Geometry: final body of the model. Coordinates: model frame, mm. Give positions to 0.01 mm unless a question says otherwise; leave off trailing zeros. Write each loop counter-clockwise with the first axis right and the second up, starting at its lowest first coordinate (ties: lowest second). Pieces come first, ordered by that corner, then holes.
Q1. Pin query (flat end, axial travel): pin 1 (3 mm diameter, centred on x = 216.51, y = 75, fed in from +Z); pin 2 (1 mm diameter, centred on y = 81, z = 48, fed in from +X). Return the tip coordinate at first contact, or that it passes through.
Q2. Line query: L1, parallel to Y at x = 215, z = 46.55; L2, parallel to X at y = 75.5, z = 47.15; L3, parallel to Y at x = 207, z = 47. Output: solid intervals per line, ascending.
Q3. Draft query along X for faces 1 (the face through (234.19, 72.19, 47.3)), 2 (the face through (215.49, 76.6, 47.3)), 3 (the face through (244.56, 39.81, 47.3)). Return one class per face: pulls with the +X half, pulls with the -X half, needs draft (parallel to the pull), parting line crosses it, or undercut.
Q4. Cut plane B-B on y = 56. Return the cut outline in (x, z), plus the area to 3 significant figures.
Q5. Cut plane C-C on x = 209. Return the cut outline in (y, z), plus the area to 3 significant figures.
```python
from build123d import *

# Parameters (mm, degrees)
ESQUISSE1_R        = 1.902389191
BOSS_EXTRU_1_DEPTH = 3


with BuildPart() as part:
    # Esquisse1 → Boss.-Extru.1 (new body)
    with BuildSketch(Plane(origin=(0, 0, 48.781012584), x_dir=(-1, 0, 0), z_dir=(0, 0, -1))):
        with BuildLine():
            Line((-246.569633903, 56.844858091), (-221.455699093, 87.978285117))
            Line((-221.455699093, 87.978285117), (-202.775642878, 72.909924232))
            Line((-202.775642878, 72.909924232), (-227.889577687, 41.776497206))
            ThreePointArc((-227.889577687, 41.776497206), (-244.763786238, 39.970649541), (-246.569633903, 56.844858091))
        make_face()
        with Locations((-237.229605795, 49.310677648)):
            Circle(ESQUISSE1_R, mode=Mode.SUBTRACT)
        with Locations((-216.510609577, 74.995754945)):
            Circle(ESQUISSE1_R, mode=Mode.SUBTRACT)
    extrude(amount=BOSS_EXTRU_1_DEPTH)


solid = part.part
```
Data:
1. pin 1: passes through
1. pin 2: stops at x = 227.49
2. L1: y = 57.76 to 73.84, 76.15 to 82.77
2. L2: x = 205.99 to 214.68, 218.34 to 231.52
2. L3: y = 67.67 to 76.32
3. face 1: pulls with the +X half
3. face 2: undercut
3. face 3: parting line crosses it
4. outline: (216.42, 45.78) - (247.19, 45.78) - (247.19, 48.78) - (216.42, 48.78) - close
4. area: 92.3 mm2
5. outline: (65.19, 45.78) - (77.93, 45.78) - (77.93, 48.78) - (65.19, 48.78) - close
5. area: 38.2 mm2
